Read the model definition and answer for the solid it produces. Units are mm, in the model's axes. A direction names the side the tool comes from. Give positions to 0.01 mm unless a question says otherwise; leave off trailing zeros. Loops run counter-clockwise (first coordinate to the right, second up) from the corner with the lowest first, then second, coordinate; pieces in that order, holes last.
(1) Which of the six approach directions +Z, -Z, +X, -X, +Y, -Y give full straight-line access (tool end or side, diameter ignored) to faces 4 (the face through (6.5, -3.9, -3.082)), 5 (the face through (11, 11, -11)), 6 (the face through (15.2, 12, -7)), 7 (the face through (12.5, -3.9, -10.745))?
(2) Find section A-A, the plane y = -3.5. Write down the section's boundary in (x, z).
(3) Find section C-C, the plane x = 14.25. Write down the section's boundary in (y, z), then the cut area to 3 significant figures.
(4) Straight lines are drawn through the part: probe 1 along X at (y, z) = (-3.25, -3.25); probe 2 along Y at (x, z) = (5.25, -0.5); probe 3 along Y at (x, z) = (8, -3.25). For each, find the intervals that lie inside material, in ascending order.
(5) Each of these flat-tipped pins is pushed along its axis until it touches: P1, Ø6, axis at x = 7, y = 1, coming from the +Z side; P2, Ø0.8, axis at x = 12.5, y = -3, coming from the -Z side (3 decimals); P3, Ø7, axis at x = 7.5, z = -6.5, coming from the +Y side; P4, Ø6, axis at y = -5, z = -6.5, coming from the -X side. Where does it stop, or does it pass through?
(6) Find section B-B, the plane z = -6.75. State how many separate pieces and enclosed holes the cut face has, then the cut area to 3 significant figures.
(7) Determine the mould class of faces 1 (the face through (0, 5, -7)), 2 (the face through (12, -4, -7)), 3 (the face through (12.5, -3.9, -3.082)) for opening direction X: pulls with the +X half, pulls with the -X half, needs draft (parallel to the pull), parting line crosses it, or undercut.
(8) Find section D-D, the plane z = -5. Write down the section's boundary in (x, y), then the cut area to 3 significant figures.
```python
from build123d import *

# Parameters (mm, degrees)
SKETCH1_W           = 17
SKETCH1_H           = 14
BOSS_EXTRUDE1_DEPTH = 10
SKETCH2_W           = 13.4
SKETCH2_H           = 8
BOSS_EXTRUDE2_DEPTH = 5
CUT_EXTRUDE4_START  = -8
CUT_EXTRUDE4_DEPTH  = 8
SKETCH4_W           = 1
SKETCH4_H           = 7.663229465
BOSS_EXTRUDE3_DEPTH = 8
SKETCH5_R           = 1
CUT_EXTRUDE5_DEPTH  = 25.289915603


# Read off the part's stored shape, not the designer's step: Cut-Extrude4
with BuildPart() as part:
    # Sketch1 → Boss-Extrude1 (new body)
    with BuildSketch(Plane(origin=(0, 0, 0), x_dir=(1, 0, 0), z_dir=(0, 1, 0))):
        with Locations((8.5, 7)):
            Rectangle(SKETCH1_W, SKETCH1_H)
    extrude(amount=BOSS_EXTRUDE1_DEPTH)

    # Sketch2 → Boss-Extrude2 (add)
    with BuildSketch(Plane(origin=(0, 10, 0), x_dir=(1, 0, 0), z_dir=(0, 1, 0))):
        with Locations((8.5, 7)):
            Rectangle(SKETCH2_W, SKETCH2_H)
    extrude(amount=BOSS_EXTRUDE2_DEPTH)

    # Cut-Extrude4 outline → Cut-Extrude4 (cut)
    with BuildSketch(Plane.XY.offset(-3).offset(CUT_EXTRUDE4_START)):
        with BuildLine():
            Line((1.8, 15), (1.8, 10))
            ThreePointArc((1.8, 10), (8.708594461, 11.940966845), (15.2, 15))
            Line((15.2, 15), (1.8, 15))
        make_face()
    extrude(amount=CUT_EXTRUDE4_DEPTH, mode=Mode.SUBTRACT)

    # Sketch4 → Boss-Extrude3 (add)
    with BuildSketch(Plane.XZ):
        with Locations((6.5, -6.913355446)):
            Rectangle(SKETCH4_W, SKETCH4_H)
        with Locations((12.5, -6.913355446)):
            Rectangle(SKETCH4_W, SKETCH4_H)
    extrude(amount=BOSS_EXTRUDE3_DEPTH)

    # Sketch5 → Cut-Extrude5 (cut, through all)
    with BuildSketch(Plane(origin=(13, 0, 0), x_dir=(0, 0, -1), z_dir=(1, 0, 0))):
        with Locations((6.913355446, -1.867470442)):
            Circle(SKETCH5_R)
        with Locations((6.913355446, -5.464189838)):
            Circle(SKETCH5_R)
    extrude(amount=-CUT_EXTRUDE5_DEPTH, mode=Mode.SUBTRACT)


solid = part.part
```
Entries:
1. face 4: +Z, +X, -X, -Y
1. face 5: -Z, +X, -X, +Y
1. face 6: +Z, -Z, +X, +Y
1. face 7: -Z, +X, -X, -Y
2. outline: (6, -10.74) - (7, -10.74) - (7, -3.08) - (6, -3.08) - close; (12, -10.74) - (13, -10.74) - (13, -3.08) - (12, -3.08) - close
3. outline: (0, -14) - (10, -14) - (10, -11) - (14.47, -11) - (14.47, -3) - (10, -3) - (10, 0) - (0, 0) - close
3. area: 176 mm2
4. probe 1: x = 6 to 7, 12 to 13
4. probe 2: y = 0 to 10
4. probe 3: y = 0 to 11.68
5. P1: stops at z = 0
5. P2: stops at z = -10.745
5. P3: stops at y = 12.87
5. P4: stops at x = 6
6. separate pieces: 5
6. enclosed holes: 0
6. area: 206 mm2
7. face 1: pulls with the -X half
7. face 2: undercut
7. face 3: needs draft
8. outline: (0, 0) - (6, 0) - (6, -8) - (7, -8) - (7, 0) - (12, 0) - (12, -8) - (13, -8) - (13, 0) - (17, 0) - (17, 10) - (15.2, 10) - (15.2, 15) arc R43.15 cw to (1.8, 10) - (0, 10) - close
8. area: 214 mm2
